from build123d import *

# Parameters (mm, degrees)
SKETCH_1_W          = 140
SKETCH_1_H          = 70
SKETCH_1_W_2        = 138
SKETCH_1_H_2        = 68
EXTRUDE_1_DEPTH     = 70
SKETCH_1_3_W        = 140
SKETCH_1_3_H        = 70
EXTRUDE_1_2_DEPTH   = 1
SKETCH_2_W          = 1
SKETCH_2_H          = 68
EXTRUDE_1_3_DEPTH   = 68
SKETCH_3_W          = 68
SKETCH_3_H          = 68
CUT_EXTRUDE_1_DEPTH = 25
SKETCH_4_W          = 1
SKETCH_4_H          = 70
EXTRUDE_2_DEPTH     = 42
SKETCH_5_R          = 5
SKETCH_5_R_2        = 3
EXTRUDE_3_DEPTH     = 20
SKETCH_6_W          = 68
SKETCH_6_H          = 1
EXTRUDE_4_DEPTH     = 41.5
SKETCH_8_R          = 1.5
CUT_EXTRUDE_2_DEPTH = 100
SKETCH_10_W         = 98
SKETCH_10_H         = 70
CUT_EXTRUDE_5_DEPTH = 1
SKETCH_11_R         = 1.5
CUT_EXTRUDE_6_DEPTH = 1.5
SKETCH_12_W         = 23.5
SKETCH_12_H         = 23.5
CUT_EXTRUDE_7_DEPTH = 28.5
SKETCH_13_R         = 5
CUT_EXTRUDE_8_DEPTH = 16.5


with BuildPart() as part:
    # Sketch 1 → Extrude 1 (new body)
    with BuildSketch(Plane.XY):
        with Locations((15.470629231, 4.392672242)):
            Rectangle(SKETCH_1_W, SKETCH_1_H)
        with Locations((15.470629231, 4.392672242)):
            Rectangle(SKETCH_1_W_2, SKETCH_1_H_2, mode=Mode.SUBTRACT)
    extrude(amount=EXTRUDE_1_DEPTH)

    # Sketch 1_3 → Extrude 1 2 (add)
    with BuildSketch(Plane.XY):
        with Locations((15.470629231, 4.392672242)):
            Rectangle(SKETCH_1_3_W, SKETCH_1_3_H)
    extrude(amount=EXTRUDE_1_2_DEPTH)

    # Sketch 2 → Extrude 1 3 (add)
    with BuildSketch(Plane.XY.offset(1)):
        with Locations((-13.029370769, 4.392672242)):
            Rectangle(SKETCH_2_W, SKETCH_2_H)
    extrude(amount=EXTRUDE_1_3_DEPTH)

    # Sketch 3 → Cut-Extrude 1 (cut)
    with BuildSketch(Plane.ZY.offset(54.529370769)):
        with Locations((35, 4.392672242)):
            Rectangle(SKETCH_3_W, SKETCH_3_H)
    extrude(amount=-CUT_EXTRUDE_1_DEPTH, mode=Mode.SUBTRACT)

    # Sketch 4 → Extrude 2 (add)
    with BuildSketch(Plane.ZY.offset(54.529370769)):
        with Locations((69.5, 4.392672242)):
            Rectangle(SKETCH_4_W, SKETCH_4_H)
    extrude(amount=-EXTRUDE_2_DEPTH)

    # Sketch 5 → Extrude 3 (add)
    with BuildSketch(Plane.ZY.offset(13.529370769)):
        with Locations(Location((35, 14.392672242, 0), (0, 0, 90))):
            Circle(SKETCH_5_R)
        with Locations(Location((35, 14.392672242, 0), (0, 0, 270))):
            Circle(SKETCH_5_R_2, mode=Mode.SUBTRACT)
    extrude(amount=EXTRUDE_3_DEPTH)

    # Sketch 6 → Extrude 4 (add)
    with BuildSketch(Plane.ZY.offset(13.529370769)):
        with Locations((35, -14.107327758)):
            Rectangle(SKETCH_6_W, SKETCH_6_H)
    extrude(amount=EXTRUDE_4_DEPTH)

    # Sketch 8 → Cut-Extrude 2 (cut, symmetric)
    with BuildSketch(Plane.XZ.offset(-38.392672242)):
        with Locations(Location((3.470629231, 66, 0), (0, 0, 90))):
            Circle(SKETCH_8_R)
        with Locations(Location((69.470629231, 66, 0), (0, 0, 90))):
            Circle(SKETCH_8_R)
    extrude(amount=CUT_EXTRUDE_2_DEPTH, both=True, mode=Mode.SUBTRACT)

    # Sketch 10 → Cut-Extrude 5 (cut)
    with BuildSketch(Plane.XY.offset(70)):
        with Locations((36.470629231, 4.392672242)):
            Rectangle(SKETCH_10_W, SKETCH_10_H)
    extrude(amount=-CUT_EXTRUDE_5_DEPTH, mode=Mode.SUBTRACT)

    # Sketch 11 → Cut-Extrude 6 (cut)
    with BuildSketch(Plane(origin=(0, -13.607327758, 0), x_dir=(1, 0, 0), z_dir=(0, 1, 0))):
        with Locations(Location((-48.938859946, -61.922756224, 0), (0, 0, 180))):
            Circle(SKETCH_11_R)
    extrude(amount=-CUT_EXTRUDE_6_DEPTH, mode=Mode.SUBTRACT)

    # Sketch 12 → Cut-Extrude 7 (cut)
    with BuildSketch(Plane(origin=(0, 39.392672242, 0), x_dir=(1, 0, 0), z_dir=(0, 1, 0))):
        with Locations((39.938426457, -36.544993355)):
            Rectangle(SKETCH_12_W, SKETCH_12_H)
    extrude(amount=-CUT_EXTRUDE_7_DEPTH, mode=Mode.SUBTRACT)

    # Sketch 13 → Cut-Extrude 8 (cut)
    with BuildSketch(Plane.ZY.offset(13.529370769)):
        with Locations(Location((49, -22.607327758, 0), (0, 0, 270))):
            Circle(SKETCH_13_R)
    extrude(amount=-CUT_EXTRUDE_8_DEPTH, mode=Mode.SUBTRACT)


solid = part.part
Verification items for the finished model (mm, model axes). A direction names the side the tool comes from. Coordinates: 2 decimals unless noted, no trailing zeros. Order: outer loops, then holes, each group sorted by start corner. A loop starts at its lowest first (then second) coordinate and runs counter-clockwise, first axis right, second up. Notation, with made-up numbers: M 67,23 L 109,23 A29 cw 109,50 Z; hole C -19,59 d1. An arc over 180 degrees is marked long. Write each question's results on one line, items separated by ' | '.
1) Section check A-A on z = 6.5. Record the cut outline in (x, y), plus the area to 4 significant figures.
Solved:
outline: M -55.03,-14.61 L -13.53,-14.61 L -13.53,-29.61 L -54.53,-29.61 L -54.53,-30.61 L 85.47,-30.61 L 85.47,39.39 L -54.53,39.39 L -54.53,38.39 L -13.53,38.39 L -13.53,-13.61 L -55.03,-13.61 Z; hole M -12.53,-29.61 L 84.47,-29.61 L 84.47,38.39 L -12.53,38.39 Z | area: 457.5 mm²
2) Gauge pin test, flat ends, axial feed: pin 1 Ø1.8 at (y, z) = (14, 36.5) entering from -X; pin 2 Ø1 at (x, z) = (32, 42.5) entering from +Y; pin 3 Ø3 at (x, y) = (46.5, 23.5) entering from +Z. Record the tip position at first contact, or that the pin passes through.
Solved:
pin 1: stops at x = -13.53 | pin 2: stops at y = -29.61 | pin 3: stops at z = 1
3) Scan lines: line 1 along Y through (x, z) = (-23, 4); line 2 along Y through (x, z) = (64, 33); line 3 along X through (y, z) = (33.5, 21.5). Record each from-to range of solid material in increasing order. Write a range as [from, to].
Solved:
line 1: y = [-30.61, -29.61], [-14.61, -13.61], [38.39, 39.39] | line 2: y = [-30.61, -29.61], [38.39, 39.39] | line 3: x = [-13.53, -12.53], [84.47, 85.47]
4) Release check for a two-part mould opening along Y. For faces 4 (the face through (85.471, 4, 34)), 5 (the face through (-33.529, 17, 37)), 6 (the face through (14, -30.607, 35)) record: pulls with the +Y half, pulls with the -Y half, needs draft (parallel to the pull), parting line crosses it, or undercut.
Solved:
face 4: needs draft | face 5: undercut | face 6: pulls with the -Y half
5) Access from +Z, -Z, +X, -X, +Y, -Y to the whole of each face (thin tool, end or side, straight path). Record for faces 1 (the face through (-34, 12, 1)), 2 (the face through (35, 5, 1)), 3 (the face through (3.02, -30.1, 67.43)).
Solved:
face 1: -X | face 2: +Z | face 3: +Y, -Y
6) Section check B-B on x = 61.5. Record the cut outline in (y, z), plus the area to 3 significant figures.
Solved:
outline: M -30.61,0 L 39.39,0 L 39.39,69 L 38.39,69 L 38.39,1 L -29.61,1 L -29.61,69 L -30.61,69 Z | area: 206 mm²
7) Section check C-C on z = 66. Give the number of separate pieces and of enclosed holes in the cut face, plus the area to 4 significant figures.
Solved:
separate pieces: 4 | enclosed holes: 0 | area: 445.5 mm²
8) Section check D-D on y = -22.5. Record the cut outline in (x, z).
Solved:
outline: M -54.53,0 L 85.47,0 L 85.47,69 L 84.47,69 L 84.47,1 L -12.53,1 L -12.53,44 L -13.53,44 L -13.53,1 L -54.53,1 Z; M -54.53,69 L -13.53,69 L -13.53,54 L -12.53,54 L -12.53,70 L -54.53,70 Z
